```python
from build123d import *

# Parameters (mm, degrees)
SKETCH1_R           = 17.5
SKETCH1_R_2         = 10
BOSS_EXTRUDE1_DEPTH = 20
SKETCH2_R           = 15
SKETCH2_R_2         = 10
BOSS_EXTRUDE2_DEPTH = 70


with BuildPart() as part:
    # Sketch1 → Boss-Extrude1 (new body)
    with BuildSketch(Plane.XY):
        with BuildLine():
            Line((0, 138), (0, 0))
            Line((0, 0), (522.5, 0))
            Line((522.5, 0), (522.5, 60))
            Line((522.5, 60), (374.6494, 86.07005))
            Line((374.6494, 86.07005), (244.94, 310.733321))
            ThreePointArc((244.94, 310.733321), (200.912249, 330.84879), (153, 337.740187))
            Line((153, 337.740187), (153, 281.918848))
            Line((153, 281.918848), (4.984782, 149.16671))
            ThreePointArc((4.984782, 149.16671), (1.302769, 144.114398), (0, 138))
        make_face()
        with Locations((153, 167.740187)):
            Circle(SKETCH1_R, mode=Mode.SUBTRACT)
        with Locations((15, 138)):
            Circle(SKETCH1_R_2, mode=Mode.SUBTRACT)
    extrude(amount=BOSS_EXTRUDE1_DEPTH)

    # Sketch2 → Boss-Extrude2 (add)
    with BuildSketch(Plane.XY.offset(20)):
        with Locations((15, 138)):
            Circle(SKETCH2_R)
        with Locations((15, 138)):
            Circle(SKETCH2_R_2, mode=Mode.SUBTRACT)
    extrude(amount=-BOSS_EXTRUDE2_DEPTH)


solid = part.part
```
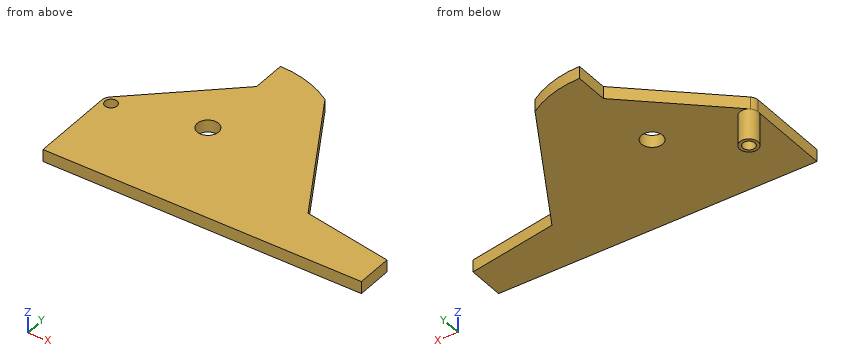
Geometry check sheet. Reference: the model listing, model coordinates, mm. Round coordinates to 2 decimals unless told otherwise and drop trailing zeros. Write each loop counter-clockwise with the first axis right and the second up, starting at its lowest first coordinate (ties: lowest second). Pieces come first, ordered by that corner, then holes. Notation, with made-up numbers: (47, 51) -> (54, 51) arc R22 ccw to (54, 66) -> close; hole circle Ø2 at (56.25, 34.5). An arc over 180 degrees is marked (long way). Put each result on its own line as item: value.
1) Cross-section at D-D, the plane y = 80.5. Enter the section's corners in (x, z).
Recorded:
outline: (0, 0) -> (406.24, 0) -> (406.24, 20) -> (0, 20) -> close
2) Cross-section at B-B, the plane z = -15.5. Enter the section's corners in (x, y), plus the area to 3 significant figures.
Recorded:
outline: circle Ø30 at (15, 138); hole circle Ø20 at (15, 138)
area: 393 mm2
3) Depth check by flat-ended pin: P1, Ø16, axis at y = 302.5, z = 13.5, coming from the -X side. Enter the tip coordinate at first touch or a pass-through.
Recorded:
P1: stops at x = 153
4) Cross-section at A-A, the plane x = 15. Enter the section's corners in (y, z).
Recorded:
outline: (0, 0) -> (123, 0) -> (123, -50) -> (128, -50) -> (128, 20) -> (0, 20) -> close; (148, -50) -> (153, -50) -> (153, 0) -> (158.15, 0) -> (158.15, 20) -> (148, 20) -> close
5) Thickness scan on probe 1 along Y at (x, z) = (15, -17.5); probe 2 along Z at (x, y) = (285, 187); probe 3 along Y at (x, z) = (15, 13.25). Record the ranges inside material, lowest first. Write a range as from..to.
Recorded:
probe 1: y = 123..128, 148..153
probe 2: z = 0..20
probe 3: y = 0..128, 148..158.15
6) Cross-section at C-C, the plane z = 14.5. Enter the section's corners in (x, y).
Recorded:
outline: (0, 0) -> (522.5, 0) -> (522.5, 60) -> (374.65, 86.07) -> (244.94, 310.73) arc R170 ccw to (153, 337.74) -> (153, 281.92) -> (4.98, 149.17) arc R15 ccw to (0, 138) -> close; hole circle Ø20 at (15, 138); hole circle Ø35 at (153, 167.74)
